Could you check a few things on this model? Use its own coordinates, in mm. Face numbers are marked on the shaded views. A direction names the side the tool comes from. Give positions to 0.01 mm unless a question says otherwise; leave off trailing zeros. Loops run counter-clockwise (first coordinate to the right, second up) from the corner with the lowest first, then second, coordinate; pieces in that order, holes last. Notation, with made-up numbers: M -29,6 L 0,6 A24 ccw 0,24 Z; hole C 11,-11 d7. An arc over 180 degrees is marked long. Return JSON: item names as keys, results as strings. Group by question number.
1. Please list where these lines run through material, in increasing order: line 1 (X direction, y = 0, z = 13.75); line 2 (X direction, y = -2.5, z = 4.5).
2. For the marked faces 4 and 5, which set-ups out of +Z, -Z, +X, -X, +Y, -Y let a thin tool reach every point of the face, with its end or its side?
3. If we section it at A-A (y = 0): Write out the boundary of the cut face in (x, z).
4. If we mould it in two halves opening along Y, with no side actions, what happens to the marked faces 1, 2 and 3? For each: +Y half, -Y half, draft (parallel to the pull), parting line (faces both ways), or undercut.
5. For pin 1 (5 mm diameter, centred on x = 0, y = 0, fed in from +Z), with a flat end and sliding along its axis, tell me the tip position at first contact or that it passes through.
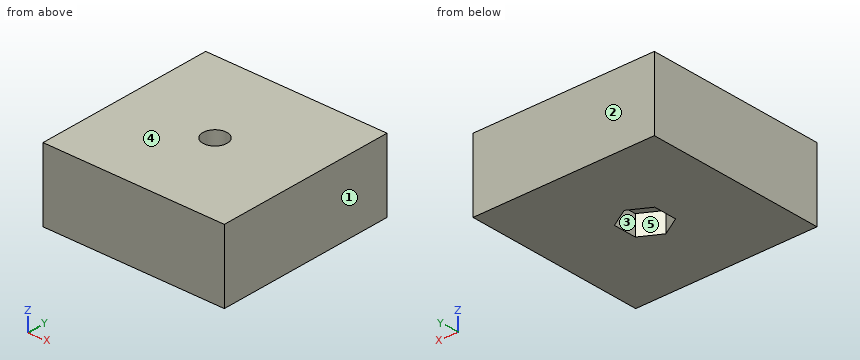
```python
from build123d import *

# Parameters (mm, degrees)
F0_W     = 45
F0_H     = 45
F1_DEPTH = 18
F2_R     = 3
F3_DEPTH = 18.001
F6_DEPTH = 5


with BuildPart() as f1:
    # F0 (on Top) → F1 (new body)
    with BuildSketch(Plane.XY):
        Rectangle(F0_W, F0_H)
    extrude(amount=F1_DEPTH)

    # F2 (on Top) → F3 (cut, through all)
    with BuildSketch(Plane.XY):
        Circle(F2_R)
    extrude(amount=F3_DEPTH, mode=Mode.SUBTRACT)

    # F5 (on face) → F6 (cut)
    with BuildSketch(Plane(origin=(0, 0, 0), x_dir=(1, 0, 0), z_dir=(0, 0, -1))):
        Polygon((5, -2.886751), (5, 2.886751), (0, 5.773503), (-5, 2.886751), (-5, -2.886751), (0, -5.773503), align=None)
    extrude(amount=-F6_DEPTH, mode=Mode.SUBTRACT)


solid = f1.part
```
Answer:
{
 "1": {"line 1": "x = -22.5 to -3, 3 to 22.5", "line 2": "x = -22.5 to -5, 5 to 22.5"},
 "2": {"face 4": "+Z, +X, -X, +Y, -Y", "face 5": "-Z"},
 "3": {"outline": "M -22.5,0 L -5,0 L -5,5 L -3,5 L -3,18 L -22.5,18 Z; M 3,5 L 5,5 L 5,0 L 22.5,0 L 22.5,18 L 3,18 Z"},
 "4": {"face 1": "draft", "face 2": "+Y half", "face 3": "undercut"},
 "5": {"pin 1": "passes through"}
}
